Input: part model. Units: mm. Frame: model coordinates. Round coordinates to 2 decimals unless told otherwise and drop trailing zeros. Write each loop counter-clockwise with the first axis right and the second up, starting at its lowest first coordinate (ties: lowest second). Pieces come first, ordered by that corner, then holes. Notation, with made-up numbers: (77, -16) -> (92, -16) arc R9 ccw to (92, -9) -> close; hole circle Ø5 at (85.25, 67.25). An arc over 180 degrees is marked (long way). Write item = value, one per line.
```python
from build123d import *

# Parameters (mm, degrees)
BOSS_EXTRUDE2_DEPTH = 400
FILLET5_R           = 0.5
SKETCH3_R           = 3
CUT_EXTRUDE2_DEPTH  = 4.5
SKETCH4_R           = 1.75
CUT_EXTRUDE3_DEPTH  = 14.5
SKETCH5_W           = 12
SKETCH5_H           = 4.057387372
CUT_EXTRUDE4_DEPTH  = 682.5
SKETCH6_W           = 13.958482149
SKETCH6_H           = 9.545138528
CUT_EXTRUDE5_DEPTH  = 50


with BuildPart() as part:
    # Sketch1 → Boss-Extrude2 (new body)
    with BuildSketch(Plane.XY):
        Polygon((0, 0), (12, 0), (12, 8.403449878), (9.5, 9.846825551), (12, 11.290201224), (12, 12), (0, 12), (0, 11.290201224), (2.5, 9.846825551), (0, 8.403449878), align=None)
    extrude(amount=BOSS_EXTRUDE2_DEPTH)

    # Fillet5
    # the kernel refuses this fillet: 0.5 mm, written as the material it adds along each edge
    with BuildSketch(Plane(origin=(2.5, 9.846825551, 0), x_dir=(-0.8660254037844382, 0.5000000000000009, 0), z_dir=(0, 0, 1)), Plane(origin=(9.5, 9.846825551, 0), x_dir=(0.8660254037844379, -0.5000000000000013, 0), z_dir=(0, 0, 1))) as fillet5_piece_1:
        with BuildLine():
            CenterArc((FILLET5_R * 1.73205080757, FILLET5_R), FILLET5_R, 150, 120)
            Line((FILLET5_R * 0.866025403784, FILLET5_R * 1.5), (0, 0))
            Line((0, 0), (FILLET5_R * 1.73205080757, 0))
        make_face()
    extrude(amount=400)
    # the kernel refuses this fillet: 0.5 mm, written as the material it takes off along each edge
    with BuildSketch(Plane(origin=(0, 8.403449878, -0.721687836), x_dir=(0, -1, 0), z_dir=(0, 0, 1))) as fillet5_2_piece_1:
        with BuildLine():
            CenterArc((FILLET5_R * 0.57735026919, FILLET5_R), FILLET5_R, 210, 60)
            Line((-FILLET5_R * 0.288675134595, FILLET5_R * 0.5), (0, 0))
            Line((0, 0), (FILLET5_R * 0.57735026919, 0))
        make_face()
    extrude(amount=401.443375673, mode=Mode.SUBTRACT)
    with BuildSketch(Plane(origin=(0, 11.290201224, -0.721687836), x_dir=(0, 1, 0), z_dir=(0, 0, 1)), Plane(origin=(12, 11.290201224, -0.721687836), x_dir=(-0.8660254037844355, -0.5000000000000052, 0), z_dir=(0, 0, 1)), Plane(origin=(12, 8.403449878, -0.721687836), x_dir=(0, -1, 0), z_dir=(0, 0, 1))) as fillet5_2_piece_2:
        with BuildLine():
            CenterArc((FILLET5_R * 0.57735026919, -FILLET5_R), FILLET5_R, 90, 60)
            Line((-FILLET5_R * 0.288675134595, -FILLET5_R * 0.5), (0, 0))
            Line((0, 0), (FILLET5_R * 0.57735026919, 0))
        make_face()
    extrude(amount=401.443375673, mode=Mode.SUBTRACT)
    with BuildSketch(Plane(origin=(0, 12, -1.25), x_dir=(1, 0, 0), z_dir=(0, 0, 1)), Plane(origin=(12, 12, -1.25), x_dir=(0, -1, 0), z_dir=(0, 0, 1))) as fillet5_2_piece_3:
        with BuildLine():
            CenterArc((FILLET5_R, -FILLET5_R), FILLET5_R, 90, 90)
            Line((0, -FILLET5_R), (0, 0))
            Line((0, 0), (FILLET5_R, 0))
        make_face()
    extrude(amount=402.5, mode=Mode.SUBTRACT)

    # Sketch3 → Cut-Extrude2 (cut)
    with BuildSketch(Plane(origin=(0, 12, 0), x_dir=(1, 0, 0), z_dir=(0, 1, 0))):
        with Locations((6, -490)):
            Circle(SKETCH3_R)
        with Locations((6, -440)):
            Circle(SKETCH3_R)
        with Locations((6, -415)):
            Circle(SKETCH3_R)
        with Locations(Location((6, -390, 0), (0, 0, 180))):
            Circle(SKETCH3_R)
        with Locations(Location((6, -365, 0), (0, 0, 180))):
            Circle(SKETCH3_R)
        with Locations(Location((6, -340, 0), (0, 0, 180))):
            Circle(SKETCH3_R)
        with Locations(Location((6, -315, 0), (0, 0, 180))):
            Circle(SKETCH3_R)
        with Locations(Location((6, -290, 0), (0, 0, 180))):
            Circle(SKETCH3_R)
        with Locations(Location((6, -265, 0), (0, 0, 180))):
            Circle(SKETCH3_R)
        with Locations(Location((6, -240, 0), (0, 0, 180))):
            Circle(SKETCH3_R)
        with Locations(Location((6, -215, 0), (0, 0, 180))):
            Circle(SKETCH3_R)
        with Locations(Location((6, -190, 0), (0, 0, 180))):
            Circle(SKETCH3_R)
        with Locations(Location((6, -165, 0), (0, 0, 180))):
            Circle(SKETCH3_R)
        with Locations(Location((6, -140, 0), (0, 0, 180))):
            Circle(SKETCH3_R)
        with Locations(Location((6, -115, 0), (0, 0, 180))):
            Circle(SKETCH3_R)
        with Locations(Location((6, -90, 0), (0, 0, 180))):
            Circle(SKETCH3_R)
        with Locations(Location((6, -65, 0), (0, 0, 180))):
            Circle(SKETCH3_R)
        with Locations(Location((6, -40, 0), (0, 0, 180))):
            Circle(SKETCH3_R)
        with Locations(Location((6, -15, 0), (0, 0, 180))):
            Circle(SKETCH3_R)
        with Locations((6, -465)):
            Circle(SKETCH3_R)
    extrude(amount=-CUT_EXTRUDE2_DEPTH, mode=Mode.SUBTRACT)

    # Sketch4 → Cut-Extrude3 (cut)
    with BuildSketch(Plane(origin=(0, 12, 0), x_dir=(1, 0, 0), z_dir=(0, 1, 0))):
        with Locations(Location((6, -15, 0), (0, 0, 180))):
            Circle(SKETCH4_R)
        with Locations(Location((6, -40, 0), (0, 0, 180))):
            Circle(SKETCH4_R)
        with Locations(Location((6, -65, 0), (0, 0, 180))):
            Circle(SKETCH4_R)
        with Locations(Location((6, -90, 0), (0, 0, 180))):
            Circle(SKETCH4_R)
        with Locations(Location((6, -115, 0), (0, 0, 180))):
            Circle(SKETCH4_R)
        with Locations(Location((6, -140, 0), (0, 0, 180))):
            Circle(SKETCH4_R)
        with Locations(Location((6, -165, 0), (0, 0, 180))):
            Circle(SKETCH4_R)
        with Locations(Location((6, -190, 0), (0, 0, 180))):
            Circle(SKETCH4_R)
        with Locations(Location((6, -215, 0), (0, 0, 180))):
            Circle(SKETCH4_R)
        with Locations(Location((6, -240, 0), (0, 0, 180))):
            Circle(SKETCH4_R)
        with Locations(Location((6, -265, 0), (0, 0, 180))):
            Circle(SKETCH4_R)
        with Locations(Location((6, -290, 0), (0, 0, 180))):
            Circle(SKETCH4_R)
        with Locations(Location((6, -315, 0), (0, 0, 180))):
            Circle(SKETCH4_R)
        with Locations(Location((6, -340, 0), (0, 0, 180))):
            Circle(SKETCH4_R)
        with Locations(Location((6, -365, 0), (0, 0, 180))):
            Circle(SKETCH4_R)
        with Locations(Location((6, -390, 0), (0, 0, 180))):
            Circle(SKETCH4_R)
        with Locations((6, -415)):
            Circle(SKETCH4_R)
        with Locations((6, -440)):
            Circle(SKETCH4_R)
        with Locations((6, -465)):
            Circle(SKETCH4_R)
        with Locations((6, -490)):
            Circle(SKETCH4_R)
    extrude(amount=-CUT_EXTRUDE3_DEPTH, mode=Mode.SUBTRACT)

    # Sketch5 → Cut-Extrude4 (cut)
    with BuildSketch(Plane(origin=(0, 0, 0), x_dir=(-1, 0, 0), z_dir=(0, 0, -1))):
        with Locations((-6, 2.028693686)):
            Rectangle(SKETCH5_W, SKETCH5_H)
    extrude(amount=-CUT_EXTRUDE4_DEPTH, mode=Mode.SUBTRACT)

    # Sketch6 → Cut-Extrude5 (cut)
    with BuildSketch(Plane.XY.offset(400)):
        with Locations((6.153953848, 7.847446167)):
            Rectangle(SKETCH6_W, SKETCH6_H)
    extrude(amount=-CUT_EXTRUDE5_DEPTH, mode=Mode.SUBTRACT)


solid = part.part
```
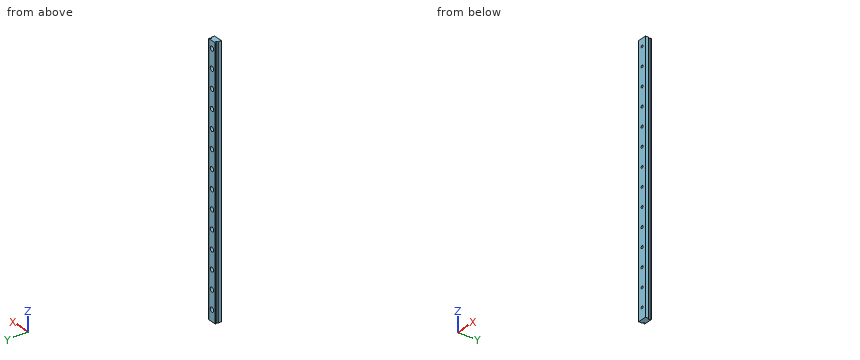
1) First-contact query: P1, Ø1, axis at y = 10, z = 164, coming from the -X side; P2, Ø1.8, axis at x = 5.5, z = 14, coming from the +Y side. Flat tips, straight axial feed; report the tip coordinate or a pass-through.
Solutions:
P1 = 1.37
P2 = 7.5
2) Cut plane A-A (z = 282). Return the cut outline in (x, y).
Solutions:
outline = (0, 4.06) -> (12, 4.06) -> (12, 8.11) arc R0.5 ccw to (11.75, 8.55) -> (10.25, 9.41) arc R0.5 cw to (10.25, 10.28) -> (11.75, 11.15) arc R0.5 ccw to (12, 11.54) arc R0.5 ccw to (11.5, 12) -> (0.5, 12) arc R0.5 ccw to (0, 11.54) arc R0.5 ccw to (0.25, 11.15) -> (1.75, 10.28) arc R0.5 cw to (1.75, 9.41) -> (0.25, 8.55) arc R0.5 ccw to (0, 8.11) -> close
3) Line query: L1, parallel to X at y = 5.2, z = 240; L2, parallel to Y at x = 11.5, z = 292.5; L3, parallel to X at y = 10.55, z = 315. Output: solid intervals per line, ascending. Write a range as from..to.
Solutions:
L1 = 0..4.25, 7.75..12
L2 = 4.06..8.69, 11..12
L3 = 1.28..3, 9..10.72
